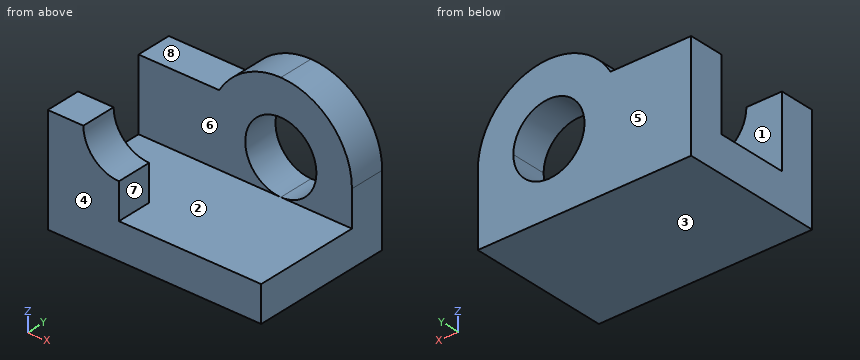
```python
from build123d import *

# Parameters (mm, degrees)
F1_DEPTH = 10
F0_W     = 20
F0_H     = 10
F2_DEPTH = 30
F0_W_2   = 60
F3_DEPTH = 40
F5_DEPTH = 10
F7_DEPTH = 10.001
F8_DEPTH = 10.001


with BuildPart() as f1:
    # F0 (on Top) → F1 (new body)
    with BuildSketch(Plane.XY):
        Polygon((20, 10), (20, 0), (60, 0), (60, 30), (0, 30), (0, 10), align=None)
    extrude(amount=F1_DEPTH)

    # F0 (on Top) → F2 (join)
    with BuildSketch(Plane.XY):
        with Locations((10, 5)):
            Rectangle(F0_W, F0_H)
    extrude(amount=F2_DEPTH)

    # F0 (on Top) → F3 (join)
    with BuildSketch(Plane.XY):
        with Locations((30, 35)):
            Rectangle(F0_W_2, F0_H)
    extrude(amount=F3_DEPTH)

    # F4 (on face) → F5 (cut, through all)
    with BuildSketch(Plane.XZ):
        with BuildLine():
            Line((20, 30), (10, 30))
            ThreePointArc((10, 30), (12.928932, 22.928932), (20, 20))
            Line((20, 20), (20, 30))
        make_face()
    extrude(amount=-F5_DEPTH, mode=Mode.SUBTRACT)

    # F6 (on face) → F7 (cut, through all)
    with BuildSketch(Plane.XZ.offset(-30)):
        with BuildLine():
            ThreePointArc((22.679492, 30), (30, 37.320508), (40, 40))
            Line((40, 40), (0, 40))
            Line((0, 40), (0, 30))
            Line((0, 30), (22.679492, 30))
        make_face()
        with BuildLine():
            ThreePointArc((40, 40), (54.142136, 34.142136), (60, 20))
            Line((60, 20), (60, 40))
            Line((60, 40), (40, 40))
        make_face()
    extrude(amount=-F7_DEPTH, mode=Mode.SUBTRACT)

    # F6 (on face) → F8 (cut, through all)
    with BuildSketch(Plane.XZ.offset(-30)):
        with BuildLine():
            ThreePointArc((50, 20), (32.928932, 27.071068), (40, 10))
            ThreePointArc((40, 10), (47.071068, 12.928932), (50, 20))
        make_face()
    extrude(amount=-F8_DEPTH, mode=Mode.SUBTRACT)


solid = f1.part
```
Input: part model. Units: mm. Frame: model coordinates. Face numbers are marked on the shaded views. A direction names the side the tool comes from. Give positions to 0.01 mm unless a question says otherwise; leave off trailing zeros. Order: outer loops, then holes, each group sorted by start corner. A loop starts at its lowest first (then second) coordinate and runs counter-clockwise, first axis right, second up.
1. Set-up query: the marked faces 5, 6, 7 and 8. Return all of +Z, -Z, +X, -X, +Y, -Y with unobstructed straight access to the full face (end or side cutting, diameter ignored); none if empty.
Computed:
face 5: +Z, -Z, +X, -X, +Y
face 6: +Z, +X, -X
face 7: +Z, +X, -Y
face 8: +Z, -X, +Y, -Y
2. Pin query (flat end, axial travel): pin 1 Ø11 at (y, z) = (7, 16.5) entering from +X; pin 2 Ø5 at (x, y) = (9.5, 5) entering from +Z; pin 3 Ø12 at (x, z) = (50.5, 30.5) entering from -Y; pin 4 Ø12 at (x, z) = (40, 20) entering from -Y. Return the tip coordinate at first contact, or that it passes through.
Computed:
pin 1: stops at x = 20
pin 2: stops at z = 30
pin 3: stops at y = 30
pin 4: passes through
3. Cut plane C-C (x = 11.5). Return loops of the section in (y, z), and give its area (3 significant figures).
Computed:
outline: (0, 0) - (40, 0) - (40, 30) - (30, 30) - (30, 10) - (10, 10) - (10, 24.73) - (0, 24.73) - close
area: 747 mm2
4. Cut plane B-B (y = 35). Return loops of the section in (x, z).
Computed:
outline: (0, 0) - (60, 0) - (60, 20) arc R20 ccw to (40, 40) arc R20 ccw to (22.68, 30) - (0, 30) - close; hole circle Ø20 at (40, 20)
5. Cut plane D-D (y = 17). Return loops of the section in (x, z).
Computed:
outline: (0, 0) - (60, 0) - (60, 10) - (0, 10) - close
6. Line query: probe 1 along X at (y, z) = (35.25, 20); probe 2 along Z at (x, y) = (40, 34). Output: solid intervals per line, ascending.
Computed:
probe 1: x = 0 to 30, 50 to 60
probe 2: z = 0 to 10, 30 to 40
7. Draft query along Y for the marked faces 1, 2, 3 and 4. Return one class per face: released by +Y, released by -Y, zero draft, split by the parting line, or undercut.
Computed:
face 1: undercut
face 2: undercut
face 3: zero draft
face 4: released by -Y
8. Cut plane A-A (x = 35.5). Return loops of the section in (y, z), and give its area (3 significant figures).
Computed:
outline: (0, 0) - (40, 0) - (40, 11.07) - (30, 11.07) - (30, 10) - (0, 10) - close; (30, 28.93) - (40, 28.93) - (40, 39.49) - (30, 39.49) - close
area: 516 mm2
